```python
from build123d import *

# Parameters (mm, degrees)
SCHIZZO1_W                   = 420
SCHIZZO1_H                   = 43.9
PIASTRABASE_DEPTH            = 2
SCHIZZO2_R                   = 9
SCHIZZO2_R_2                 = 1.75
FORODESTRO_DEPTH             = 212.153504588
INTAGLIOINFERIORE_DEPTH      = 212.153504588
INTAGLIOSUPERIORE_DEPTH      = 212.153504588
ESTRUSIONE_ESTRUSIONE1_DEPTH = 2
RACCORDO2_R                  = 10
RACCORDO3_R                  = 10
RACCORDO2_OF_SPECCHIA1_R     = 10
RACCORDO3_OF_SPECCHIA1_R     = 10


with BuildPart() as part:
    # Schizzo1 → PiastraBase (new body)
    with BuildSketch(Plane.XY):
        Rectangle(SCHIZZO1_W, SCHIZZO1_H)
    extrude(amount=PIASTRABASE_DEPTH)

    # Schizzo2 → ForoDestro (cut, through all)
    with BuildSketch(Plane(origin=(0, 0, 0), x_dir=(-1, 0, 0), z_dir=(0, 0, -1))):
        with Locations((-174.166666667, 3.05)):
            Circle(SCHIZZO2_R)
        with Locations((-193, 19.45)):
            Circle(SCHIZZO2_R_2)
        with Locations((-117, 19.45)):
            Circle(SCHIZZO2_R_2)
    forodestro = extrude(amount=-FORODESTRO_DEPTH, mode=Mode.SUBTRACT)

    # ForoSinistro: ForoDestro across plane
    add(forodestro.mirror(Plane(origin=(0, 0, 0), x_dir=(0, 0, 1), z_dir=(1, 0, 0))), mode=Mode.SUBTRACT)

    # Schizzo3 → IntaglioInferiore (cut, through all)
    with BuildSketch(Plane(origin=(0, 0, 0), x_dir=(-1, 0, 0), z_dir=(0, 0, -1))):
        Polygon((-105, -21.95), (-105, -20.45), (-87.5, -20.45), (-87.5, -11.95), (-82.5, -11.95), (-82.5, -20.45), (82.5, -20.45), (82.5, -11.95), (87.5, -11.95), (87.5, -20.45), (105, -20.45), (105, -21.95), align=None)
    extrude(amount=-INTAGLIOINFERIORE_DEPTH, mode=Mode.SUBTRACT)

    # Schizzo4 → IntaglioSuperiore (cut, through all)
    with BuildSketch(Plane(origin=(0, 0, 0), x_dir=(-1, 0, 0), z_dir=(0, 0, -1))):
        Polygon((-105, 21.95), (-104.999999109, 3.05), (-82.5, 3.05), (-82.5, -20.45), (82.5, -20.45), (82.5, 3.05), (104.999999109, 3.05), (105, 21.95), align=None)
    extrude(amount=-INTAGLIOSUPERIORE_DEPTH, mode=Mode.SUBTRACT)


with BuildPart() as intagliosuperiore_piece_1:
    # of the separate pieces the step leaves, piece 1, a body of its own (intagliosuperiore_pieces)
    add(part.part.solids().sort_by_distance((-210, 21.95, 0))[0])


with BuildPart() as intagliosuperiore_piece_2:
    # of the separate pieces the step leaves, piece 2, a body of its own (intagliosuperiore_pieces)
    add(part.part.solids().sort_by_distance((210, -21.95, 0))[0])

    # Schizzo5 → Estrusione-Estrusione1 (add)
    with BuildSketch(Plane(origin=(0, 0, 0), x_dir=(-1, 0, 0), z_dir=(0, 0, -1))):
        Polygon((-82.5, 3.05), (-82.5, 19.55), (0, 31.95), (0, 46.95), (-2, 46.95), (-2, 49.95), (-92.5, 21.55), (-97.5, 16.05), (-101.5, 3.05), align=None)
    estrusione_estrusione1 = extrude(amount=-ESTRUSIONE_ESTRUSIONE1_DEPTH)

    # Raccordo2
    raccordo2_edges = [intagliosuperiore_piece_2.edges().sort_by_distance(p)[0] for p in [
        (82.5, 19.55, 1),
    ]]
    fillet(raccordo2_edges, radius=RACCORDO2_R)

    # Raccordo3
    raccordo3_edges = [intagliosuperiore_piece_2.edges().sort_by_distance(p)[0] for p in [
        (92.5, 21.55, 1),
        (97.5, 16.05, 1),
    ]]
    fillet(raccordo3_edges, radius=RACCORDO3_R)

    # Specchia1: Estrusione-Estrusione1 across plane
    add(estrusione_estrusione1.mirror(Plane(origin=(0, 0, 0), x_dir=(0, 0, 1), z_dir=(1, 0, 0))))

    # Raccordo2 of Specchia1
    raccordo2_of_specchia1_edges = [intagliosuperiore_piece_2.edges().sort_by_distance(p)[0] for p in [
        (-82.5, 19.55, 1),
    ]]
    fillet(raccordo2_of_specchia1_edges, radius=RACCORDO2_OF_SPECCHIA1_R)

    # Raccordo3 of Specchia1
    raccordo3_of_specchia1_edges = [intagliosuperiore_piece_2.edges().sort_by_distance(p)[0] for p in [
        (-92.5, 21.55, 1),
        (-97.5, 16.05, 1),
    ]]
    fillet(raccordo3_of_specchia1_edges, radius=RACCORDO3_OF_SPECCHIA1_R)

    # Abbina1: union IntaglioSuperiore piece 1
    add(intagliosuperiore_piece_1.part)


solid = intagliosuperiore_piece_2.part
```
Build history of the part. All positions in model axes, mm. A direction names the side the tool comes from. Round coordinates to 2 decimals unless told otherwise and drop trailing zeros. Order: outer loops, then holes, each group sorted by start corner. A loop starts at its lowest first (then second) coordinate and runs counter-clockwise, first axis right, second up. Notation, with made-up numbers: (-24, 73.25) - (-16, 73.25) arc R25 cw to (-16, 100.25) - close; hole circle Ø9 at (-5.75, 44). An arc over 180 degrees is marked (long way). Use a Markdown table: item, result.
1) Tool access for faces 1 (the face through (-80.14, 17.39, 1.01)), 2 (the face through (183.158, 3.446, 0.986)): list every direction of +Z, -Z, +X, -X, +Y, -Y with a clear straight run to the whole face (end or side of a thin tool).
Recorded:
| item | result |
|---|---|
| face 1 | +Z, -Z, -Y |
| face 2 | +Z, -Z |
2) Saw through at A-A on x = -169.5. Write the cut outline in (y, z).
Recorded:
| item | result |
|---|---|
| outline | (-21.95, 0) - (-4.65, 0) - (-4.65, 2) - (-21.95, 2) - close; (10.75, 0) - (21.95, 0) - (21.95, 2) - (10.75, 2) - close |
3) Saw through at C-C on y = 37. Write the cut outline in (x, z).
Recorded:
| item | result |
|---|---|
| outline | (-43.27, 0) - (43.27, 0) - (43.27, 2) - (-43.27, 2) - close |
4) Wall check: L1, parallel to Y at x = -117, z = 1.05; L2, parallel to Y at x = 175, z = 1.7; L3, parallel to X at y = 12.5, z = 0.2. Give the ranges that are in metal, low to high.
Recorded:
| item | result |
|---|---|
| L1 | y = -21.95 to 17.7, 21.2 to 21.95 |
| L2 | y = -21.95 to -5.91, 12.01 to 21.95 |
| L3 | x = -210 to -105, -98.59 to -82.38, 82.38 to 98.59, 105 to 210 |
5) Saw through at B-B on z = 0.6. Give the number of separate pieces and of enclosed holes in the cut face, and give its area (3 significant figures).
Recorded:
| item | result |
|---|---|
| separate pieces | 1 |
| enclosed holes | 6 |
| area | 12,200 mm² |
6) Saw through at D-D on x = -63. Write the cut outline in (y, z).
Recorded:
| item | result |
|---|---|
| outline | (22.48, 0) - (30.81, 0) - (30.81, 2) - (22.48, 2) - close |
7) Flat gauge pins, fed straight in: pin 1 Ø1 at (x, z) = (26, 1.5) entering from -Y; pin 2 Ø0.6 at (x, z) = (84.5, 1) entering from -Y; pin 3 Ø1 at (x, z) = (-164, 1) entering from +Y. Where does each tip first touch, or does it go through?
Recorded:
| item | result |
|---|---|
| pin 1 | stops at y = 27.97 |
| pin 2 | stops at y = -11.95 |
| pin 3 | stops at y = 21.95 |
